from build123d import *

# Parameters (mm, degrees)
SKETCH1_R           = 3.175
BOSS_EXTRUDE1_DEPTH = 22.9108
SKETCH2_R           = 3.175
BOSS_EXTRUDE2_DEPTH = 5.588
BOSS_EXTRUDE3_REACH = 318.687


with BuildPart() as part:
    # Sketch1 → Boss-Extrude1 (new body)
    with BuildSketch(Plane.XY):
        Polygon((-279.480965909, 265.178996639), (-302.009381101, 261.299549651), (-298.138391254, 238.820246093), (-275.609976062, 242.699693081), align=None)
        with Locations(Location((-285, 257.808220008, 0), (0, 0, 90))):
            Circle(SKETCH1_R, mode=Mode.SUBTRACT)
    extrude(amount=BOSS_EXTRUDE1_DEPTH)

    # Sketch2 → Boss-Extrude2 (add)
    with BuildSketch(Plane(origin=(0, 235.555558992, -22.588757095), x_dir=(1, 0, 0), z_dir=(0, 0.9954334818448494, -0.09545775621833992))):
        Polygon((-301.340789499, 1.892568588), (-307.73958618, -66.388261818), (-286.2437692, -68.40269781), (-279.844972519, -0.121867404), align=None)
        with Locations(Location((-291.422354653, -7.965868164, 0), (0, 0, 270))):
            Circle(SKETCH2_R, mode=Mode.SUBTRACT)
        with Locations(Location((-296.162204047, -58.544261058, 0), (0, 0, 270))):
            Circle(SKETCH2_R, mode=Mode.SUBTRACT)
    extrude(amount=-BOSS_EXTRUDE2_DEPTH)

    # Boss-Extrude3: up to this face of the body (flat: up to its plane)
    boss_extrude3_end = Plane(part.part.faces().sort_by_distance((-286.17802659, 240.879849499, 10.873584724))[0])
    # Sketch4 → Boss-Extrude3 (add, up to the picked face)
    with BuildSketch(Plane(origin=(0, 235.555558992, -22.588757095), x_dir=(1, 0, 0), z_dir=(0, 0.9954334818448495, -0.09545775621833982)), mode=Mode.PRIVATE) as boss_extrude3_sk1:
        Polygon((-291.759134886, -45.708284808), (-275.609976062, -45.973745552), (-275.609976062, -23.167568136), (-298.138391254, -22.797244832), (-298.138391254, -34.200333539), align=None)
    boss_extrude3_tool1 = split(extrude(boss_extrude3_sk1.sketch, amount=BOSS_EXTRUDE3_REACH, mode=Mode.PRIVATE), bisect_by=boss_extrude3_end, keep=Keep.BOTH, mode=Mode.PRIVATE)
    add(boss_extrude3_tool1.solids().sort_by(Axis((-286.178027, 238.783728, 11.074594), (0, 0.9954334818448495, -0.09545775621833982)))[0])


solid = part.part
The model under review builds one solid part; all positions refer to its coordinate system, in mm. A direction names the side the tool comes from. Round coordinates to 2 decimals unless told otherwise and drop trailing zeros. Loops run counter-clockwise (first coordinate to the right, second up) from the corner with the lowest first, then second, coordinate; pieces in that order, holes last. Notation, with made-up numbers: M -33,45 L 20,45 A23 cw 20,56 Z; hole C 85.5,30.5 d4. An arc over 180 degrees is marked long. Answer as CSV lines item,"result".
1. To check wall thickness, follow L1, parallel to Z at x = -279.5, y = 255.5; L2, parallel to Y at x = -285, z = 5; L3, parallel to Y at x = -285, z = 18. State the ranges of each line that lie inside material, in increasing order. Write a range as [from, to].
Outcome:
L1,"z = [0, 22.91]"
L2,"y = [232.59, 254.63], [260.98, 264.23]"
L3,"y = [233.83, 254.63], [260.98, 264.23]"
2. Insertion check: pin 1 Ø6 at (y, z) = (240.5, 28) entering from -X; pin 2 Ø4 at (x, y) = (-284, 260) entering from +Z; pin 3 Ø6 at (y, z) = (243, 31) entering from -X. Each pin has a flat end and moves straight along its axis. Give the tip position at first contact, or say it passes through.
Outcome:
pin 1,"stops at x = -306.56"
pin 2,"stops at z = 22.91"
pin 3,"stops at x = -306.76"
3. We need section A-A (x = -285). Give the boundary of the cut face in (y, z).
Outcome:
outline,"M 229.96,-22.41 L 235.52,-22.95 L 237.75,0.32 L 241.08,0 L 254.63,0 L 254.63,22.91 L 241.08,22.91 L 239.93,23.02 L 240.82,32.29 L 235.26,32.82 Z; M 260.98,0 L 264.23,0 L 264.23,22.91 L 260.98,22.91 Z"
4. We need section D-D (x = -281). Give the boundary of the cut face in (y, z), plus the area to 3 significant figures.
Outcome:
outline,"M 229.99,-22.04 L 235.56,-22.58 L 236.74,-10.2 L 231.18,-9.67 Z; M 237.76,0.38 L 241.77,0 L 264.92,0 L 264.92,22.91 L 241.77,22.91 L 239.94,23.09 Z"
area,"667 mm2"
5. We need section C-C (z = 21.5). Give the boundary of the cut face in (x, y) (3 decimals).
Outcome:
outline,"M -305.669,239.783 L -305.619,234.17 L -283.934,234.17 L -283.984,239.783 L -275.61,239.783 L -275.61,242.7 L -279.481,265.179 L -302.009,261.3 L -298.304,239.783 Z; hole C -285,257.808 d6.35"
6. For faces 1 (the face through (-289, 252, 0)), 2 (the face through (-277.52, 253.78, 11.3)), list the 3-axis set-ups (+Z, -Z, +X, -X, +Y, -Y) from which the entire face can be reached by the end or side of a thin tool; tool diameter is ignored.
Outcome:
face 1,"-Z, +X, -X, +Y"
face 2,"+Z, -Z, +X, +Y"
7. Draft analysis for pull direction X (two halves, no side actions). For faces 3 (the face through (-300.1, 250.2, 11.3)), 4 (the face through (-294.522, 233.508, -15.081)), 5 (the face through (-293.014, 238.362, 35.54)), 6 (the face through (-300.186, 238.683, 10.025)), state which applies: pulls with the +X half, pulls with the -X half, needs draft (parallel to the pull), parting line crosses it, or undercut.
Outcome:
face 3,"pulls with the -X half"
face 4,"undercut"
face 5,"undercut"
face 6,"needs draft"
8. We need section B-B (y = 259). Give the boundary of the cut face in (x, z), plus the area to 3 significant figures.
Outcome:
outline,"M -301.61,0 L -287.94,0 L -287.94,22.91 L -301.61,22.91 Z; M -282.06,0 L -278.42,0 L -278.42,22.91 L -282.06,22.91 Z"
area,"397 mm2"
